```python
from build123d import *

# Parameters (mm, degrees)
T_LE_DE_BASE_PLI_E1_DEPTH    = 108
ESQUISSE2_W                  = 60
ESQUISSE2_H                  = 10
ENL_V_MAT_EXTRU_1_DEPTH      = 131.326513036
ENL_V_MAT_EXTRU_2_DEPTH      = 10
ENL_V_MAT_EXTRU_3_DEPTH      = 3
ENL_V_MAT_EXTRU_3_DEPTH_BACK = 130.073622402
ENL_V_MAT_EXTRU_4_DEPTH      = 10
ESQUISSE6_R                  = 7
ENL_V_MAT_EXTRU_5_DEPTH      = 10


# Sheet-metal steps are written as plain solids
with BuildPart() as part:
    # Esquisse1 → Tôle de base pliée1 (new body)
    with BuildSketch(Plane.ZY):
        with BuildLine():
            Line((30, 0), (5, 0))
            ThreePointArc((5, 0), (1.464466094, 1.464466094), (0, 5))
            Line((0, 5), (0, 64))
            Line((0, 64), (-5, 64))
            Line((-5, 64), (-5, 5))
            ThreePointArc((-5, 5), (-2.071067812, -2.071067812), (5, -5))
            Line((5, -5), (30, -5))
            Line((30, -5), (30, 0))
        make_face()
    extrude(amount=T_LE_DE_BASE_PLI_E1_DEPTH)

    # Esquisse2 → Enlèv. mat.-Extru.1 (cut, through all)
    with BuildSketch(Plane.XY.offset(30)):
        with Locations((-78, 0)):
            Rectangle(ESQUISSE2_W, ESQUISSE2_H)
    extrude(amount=-ENL_V_MAT_EXTRU_1_DEPTH, mode=Mode.SUBTRACT)

    # Esquisse3 → Enlèv. mat.-Extru.2 (cut)
    with BuildSketch(Plane.XY):
        with BuildLine():
            Line((-76, 64), (-123.136026385, 64))
            Line((-123.136026385, 64), (-123.136026385, 0))
            Line((-123.136026385, 0), (-76, 0))
            ThreePointArc((-76, 0), (-108, 32), (-76, 64))
        make_face()
    extrude(amount=-ENL_V_MAT_EXTRU_2_DEPTH, mode=Mode.SUBTRACT)

    # Esquisse4 → Enlèv. mat.-Extru.3 (cut, two sides: drawn at the far end of the back side and taken through both)
    with BuildSketch(Plane.XY.offset(-ENL_V_MAT_EXTRU_3_DEPTH_BACK)):
        Polygon((172.979910748, -161.583658888), (0, 15), (-48, 64), (-220.979910748, 240.583658888), (132.187407029, 586.543480383), (526.147228524, 184.376162607), align=None)
    extrude(amount=ENL_V_MAT_EXTRU_3_DEPTH + ENL_V_MAT_EXTRU_3_DEPTH_BACK, mode=Mode.SUBTRACT)

    # Esquisse5 → Enlèv. mat.-Extru.4 (cut)
    with BuildSketch(Plane(origin=(0, 0, 0), x_dir=(1, 0, 0), z_dir=(0, 1, 0))):
        with BuildLine():
            Line((-36, -15), (-36, -21))
            ThreePointArc((-36, -21), (-39, -24), (-42, -21))
            Line((-42, -21), (-42, -15))
            ThreePointArc((-42, -15), (-39, -12), (-36, -15))
        make_face()
        with BuildLine():
            Line((-6, -15), (-6, -21))
            ThreePointArc((-6, -21), (-9, -24), (-12, -21))
            Line((-12, -21), (-12, -15))
            ThreePointArc((-12, -15), (-9, -12), (-6, -15))
        make_face()
    extrude(amount=-ENL_V_MAT_EXTRU_4_DEPTH, mode=Mode.SUBTRACT)

    # Esquisse6 → Enlèv. mat.-Extru.5 (cut)
    with BuildSketch(Plane.XY):
        with Locations((-76, 32)):
            Circle(ESQUISSE6_R)
    extrude(amount=-ENL_V_MAT_EXTRU_5_DEPTH, mode=Mode.SUBTRACT)


solid = part.part
```
Geometry check sheet. Reference: the model listing, model coordinates, mm. A direction names the side the tool comes from. Round coordinates to 2 decimals unless told otherwise and drop trailing zeros. Write each loop counter-clockwise with the first axis right and the second up, starting at its lowest first coordinate (ties: lowest second). Pieces come first, ordered by that corner, then holes. Notation, with made-up numbers: (63.25, 62) -> (113.25, 62) arc R21 ccw to (113.25, 83) -> close; hole circle Ø10 at (-29, -9). An arc over 180 degrees is marked (long way). Put each result on its own line as item: value.
1) Release check for a two-part mould opening along Z. For faces 6 (the face through (-9, -2, 12)), 7 (the face through (-65, 28, -5)), 8 (the face through (-24, -5, 17)) record: pulls with the +Z half, pulls with the -Z half, needs draft (parallel to the pull), parting line crosses it, or undercut.
Recorded:
face 6: undercut
face 7: pulls with the -Z half
face 8: needs draft
2) Cross-section at B-B, the plane x = -9. Enter the section's corners in (y, z), plus the area to 3 significant figures.
Recorded:
outline: (-5, 5) arc R10 ccw to (5, -5) -> (24.19, -5) -> (24.19, 0) -> (5, 0) arc R5 cw to (0, 5) -> (0, 12) -> (-5, 12) -> close; (-5, 24) -> (0, 24) -> (0, 30) -> (-5, 30) -> close
area: 220 mm2
3) Thickness scan on probe 1 along Y at (x, z) = (-76, -1.55); probe 2 along Z at (x, y) = (-62, 13.5). Record the ranges inside material, lowest first. Write a range as from..to.
Recorded:
probe 1: y = 5..25, 39..64
probe 2: z = -5..0
4) Depth check by flat-ended pin: P1, Ø16, axis at x = -76, y = 32, coming from the +Z side; P2, Ø5.5, axis at y = -1.5, z = 19, coming from the -X side; P3, Ø5, axis at y = 21, z = 1.5, coming from the +X side. Enter the tip coordinate at first touch or a pass-through.
Recorded:
P1: stops at z = 0
P2: stops at x = -48
P3: stops at x = -3.92
5) Cross-section at A-A, the plane z = 19. Enter the section's corners in (x, y), plus the area to 3 significant figures.
Recorded:
outline: (-48, -5) -> (-42, -5) -> (-42, 0) -> (-48, 0) -> close; (-36, -5) -> (-12, -5) -> (-12, 0) -> (-36, 0) -> close; (-6, -5) -> (0, -5) -> (0, 0) -> (-6, 0) -> close
area: 180 mm2
6) Cross-section at C-C, the plane y = 29.5. Enter the section's corners in (x, z).
Recorded:
outline: (-107.9, -5) -> (-82.54, -5) -> (-82.54, 0) -> (-107.9, 0) -> close; (-69.46, -5) -> (-14.2, -5) -> (-14.2, 0) -> (-69.46, 0) -> close
7) Access from +Z, -Z, +X, -X, +Y, -Y to the whole of each face (thin tool, end or side, straight path). Record for faces 1 (the face through (-12, -2, 18)), 2 (the face through (-71, 5, -2)), 3 (the face through (-65, 28, 0)), 4 (the face through (-24, -3, 30)), 5 (the face through (0, -2, 10)).
Recorded:
face 1: +Y, -Y
face 2: +Z, -Z, -X, -Y
face 3: +Z, +X, -X, +Y
face 4: +Z, +X, -X, +Y, -Y
face 5: +Z, -Z, +X, +Y, -Y
8) Cross-section at D-D, the plane z = 10. Enter the section's corners in (x, y), plus the area to 3 significant figures.
Recorded:
outline: (-48, -5) -> (0, -5) -> (0, 0) -> (-48, 0) -> close
area: 240 mm2
